Could you check a few things on this model? Use its own coordinates, in mm. A direction names the side the tool comes from. Give positions to 0.01 mm unless a question says otherwise; leave off trailing zeros. Loops run counter-clockwise (first coordinate to the right, second up) from the corner with the lowest first, then second, coordinate; pieces in that order, holes last. Notation, with made-up numbers: (34.5, 87.5) - (39.5, 87.5) arc R30 ccw to (39.5, 115.5) - close; hole circle Ø2 at (61.25, 28). An arc over 180 degrees is marked (long way). Use CSV: the item, a comma, the result in double quotes.
from build123d import *

# Parameters (mm, degrees)
SKETCH_1_W          = 330
SKETCH_1_H          = 80
EXTRUDE_1_DEPTH     = 2
HOLE_WIZARD_M5_1_D  = 4.2
EXTRUDE_2_DEPTH     = 150
SKETCH_6_R          = 21.213203436
CUT_EXTRUDE_1_DEPTH = 280


with BuildPart() as part:
    # 草图1 → 凸台-拉伸1 (new body)
    with BuildSketch(Plane.XY):
        Rectangle(SKETCH_1_W, SKETCH_1_H)
    extrude(amount=EXTRUDE_1_DEPTH)

    # M5 螺纹孔1 (through all)
    with Locations(Plane.XY.offset(2)):
        with Locations((-155, 32), (-155, -32), (155, 32), (155, -32)):
            Hole(HOLE_WIZARD_M5_1_D / 2)

    # 草图5 → 凸台-拉伸2 (add, symmetric)
    with BuildSketch(Plane(origin=(0, 0, 0), x_dir=(0, 0, -1), z_dir=(1, 0, 0))):
        Polygon((0, 25), (0, -25), (50, 25), align=None)
    extrude(amount=EXTRUDE_2_DEPTH, both=True)

    # 草图6 → 切除-拉伸1 (cut)
    with BuildSketch(Plane(origin=(140, 0, 0), x_dir=(0, 0, -1), z_dir=(1, 0, 0))):
        with Locations((25, 0)):
            Circle(SKETCH_6_R)
    extrude(amount=-CUT_EXTRUDE_1_DEPTH, mode=Mode.SUBTRACT)


solid = part.part
1) I'm going to push flat-ended pins straight in: P1, Ø25, axis at x = -61.5, z = -25, coming from the +Y side; P2, Ø1.5, axis at x = 95.5, z = -19.5, coming from the -Y side; P3, Ø5, axis at x = -62, z = -24.5, coming from the -Y side; P4, Ø6.5, axis at x = 155, y = -32, coming from the +Z side. Where does each tip first touch, or does it pass through?
Answer below:
P1,"stops at y = 25"
P2,"stops at y = 20.27"
P3,"stops at y = 21"
P4,"stops at z = 2"
2) Suppose I cut it at D-D (y = 0). Please give me the cut outline in (x, z), plus the area to 3 significant figures.
Answer below:
outline,"(-165, 0) - (-150, 0) - (-150, -25) - (-140, -25) - (-140, -3.79) - (140, -3.79) - (140, -25) - (150, -25) - (150, 0) - (165, 0) - (165, 2) - (-165, 2) - close"
area,"2,220 mm2"
3) Suppose I cut it at A-A (y = -20.5). Please give me the cut outline in (x, z), plus the area to 3 significant figures.
Answer below:
outline,"(-165, 0) - (-150, 0) - (-150, -4.5) - (150, -4.5) - (150, 0) - (165, 0) - (165, 2) - (-165, 2) - close"
area,"2,010 mm2"
4) We'd pull the mould along Y, two halves only. Please class faces 1 (the flat face through (2, 25, -25)), 2 (the cylindrical face through (2, 15, -10)), 3 (the flat face through (-150, 6, -19)), 4 (the flat face through (2, 16, -41)): +Y half, -Y half, draft (parallel to the pull), parting line (faces both ways), or undercut.
Answer below:
face 1,"+Y half"
face 2,"undercut"
face 3,"draft"
face 4,"-Y half"
5) I need wall thicknesses on line 1 along Y through (x, z) = (-155, 0.4); line 2 along X through (y, z) = (-7.5, -8.5); line 3 along Z through (x, y) = (32, -33.5). Which ranges of each line are inside material? Lowest first, please.
Answer below:
line 1,"y = -40 to -34.1, -29.9 to 29.9, 34.1 to 40"
line 2,"x = -150 to -140, 140 to 150"
line 3,"z = 0 to 2"
6) Suppose I cut it at C-C (x = -10.5). Please give me the cut outline in (y, z).
Answer below:
outline,"(-40, 0) - (-25, 0) - (-15, -10) arc R21.21 cw to (15, -40) - (25, -50) - (25, 0) - (40, 0) - (40, 2) - (-40, 2) - close"
7) Suppose I cut it at B-B (z = -25). Please give me the cut outline in (x, y), plus the area to 3 significant figures.
Answer below:
outline,"(-150, 0) - (-140, 0) - (-140, 21.21) - (140, 21.21) - (140, 0) - (150, 0) - (150, 25) - (-150, 25) - close"
area,"1,560 mm2"
8) Which directions (+Z, -Z, +X, -X, +Y, -Y) give clear straight access to the entire face, cutting with the end or side of a thin tool? Please do faces 5 (the flat face through (-2, 1, 2)), 6 (the flat face through (-140, 7, -18)), 7 (the flat face through (150, 6, -19)).
Answer below:
face 5,"+Z, +X, -X, +Y, -Y"
face 6,"none"
face 7,"-Z, +X, +Y, -Y"
